Can you work these out from the model? Positions are in its coordinate system, mm. Face numbers are marked on the shaded views. A direction names the side the tool comes from. Coordinates: 2 decimals unless noted, no trailing zeros. Loops run counter-clockwise (first coordinate to the right, second up) from the corner with the lowest first, then second, coordinate; pieces in that order, holes last. Notation, with made-up numbers: M 35.5,24.25 L 40.5,24.25 A9 ccw 40.5,34.25 Z; hole C -19.5,85 d6. An arc over 180 degrees is marked long. Answer as a JSON object with one key per item and string values. Group by question number.
Item 1: If I drill on line 1 (Y direction, x = 8, z = -21) (3 decimals); line 2 (Z direction, x = 12, y = 2) (3 decimals), over which ranges is the centre line in solid material (lowest first)?
Item 2: Suppose I cut it at A-A (x = 14). Count the separate pieces of the cut face and the enclosed holes in it, then the cut area to 3 significant figures.
Item 3: I'm going to push flat-ended pins straight in: pin 1 Ø6 at (x, z) = (7.5, -3.5) entering from +Y (3 decimals); pin 2 Ø7.5 at (x, y) = (12.5, 22) entering from -Z; pin 3 Ø4.5 at (x, y) = (13.26, 19.76) entering from -Z. Where does each tip first touch, or does it pass through?
Item 4: Suppose I cut it at C-C (z = -16.5). Write out the boundary of the cut face in (x, y) (3 decimals).
Item 5: Which directions (+Z, -Z, +X, -X, +Y, -Y) give clear straight access to the entire face, cutting with the end or side of a thin tool? Please do the marked faces 1 and 2.
Item 6: Suppose I cut it at D-D (z = -2). Write out the boundary of the cut face in (x, y) (3 decimals).
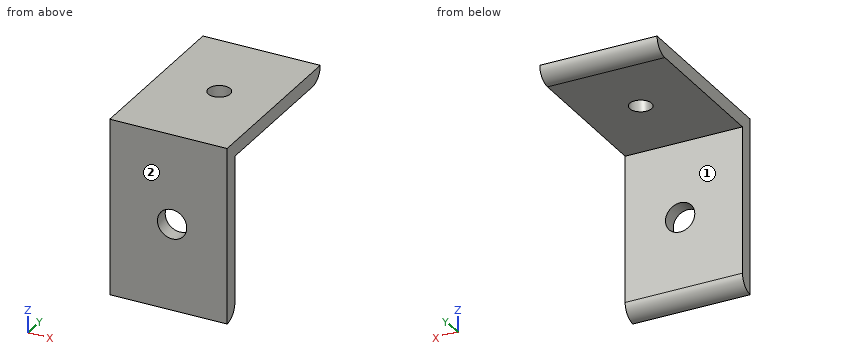
Autodesk Inventor part; units mm, degrees
ref_plane "YZ Plane" through (0, 0, 0) normal (1, 0, 0) x (0, 1, 0)
ref_plane "XZ Plane" through (0, 0, 0) normal (0, 1, 0) x (-1, 0, 0)
ref_plane "XY Plane" through (0, 0, 0) normal (0, 0, 1) x (1, 0, 0)
sketch "Sketch1" plane through (0, 0, 0) normal (0, 0, 1) x (1, 0, 0)
  line L0 (0, 0) -> (25.4, 0)
  line L1 (25.4, 0) -> (25.4, 38.1)
  line L2 (25.4, 38.1) -> (0, 38.1)
  line L3 (0, 38.1) -> (0, 0)
  dimension "d0" = 25.4
  dimension "d1" = 38.1
extrude "Extrusion1" add sketch "Sketch1" along normal blind 3.175
fillet "Fillet1" radius 3.175 1 edges at (12.7, 38.1, 0)
sketch "Sketch2" plane through (0, 0, 0) normal (0, 0, -1) x (-1, 0, 0)
  line L0 (0, 0) -> (-25.4, 0)
  line L1 (0, 38.1) -> (0, 0)
  line L2 (-25.4, 0) -> (0, 0)
  line L3 (0, 0) -> (0, 3.175)
  line L4 (0, 3.175) -> (-25.4, 3.175)
  line L5 (-25.4, 3.175) -> (-25.4, 0)
  dimension "d5" = 3.175
extrude "Extrusion2" add sketch "Sketch2" along normal blind 34.925
fillet "Fillet2" radius 3.175 1 edges at (12.7, 3.175, -34.925)
hole "Hole1" at (13.4954, 3.175, -16.2632) direction (0, -1, 0) diameter 6.35 depth 25.4 tip angle 118
hole "Hole2" at (13.2558, 19.7589, 0) direction (0, 0, 1) diameter 4.7625 depth 25.4 tip angle 118
properties part number "Brackket"
From the geometry:
{
 "1": {"line 1": "0 to 3.175", "line 2": "-34.216 to -19.064, -13.462 to 3.175"},
 "2": {"separate pieces": "3", "enclosed holes": "0", "area": "193 mm2"},
 "3": {"pin 1": "y = 3.175", "pin 2": "z = 0", "pin 3": "through"},
 "4": {"outline": "M 0,0 L 10.329,0 L 10.329,3.175 L 0,3.175 Z; M 16.662,0 L 25.4,0 L 25.4,3.175 L 16.662,3.175 Z"},
 "5": {"face 1": "-Z, +X, -X, +Y", "face 2": "+Z, -Z, +X, -X, -Y"},
 "6": {"outline": "M 0,0 L 25.4,0 L 25.4,3.175 L 0,3.175 Z"}
}
